Read the model definition and answer for the solid it produces. Units are mm, in the model's axes. Face numbers are marked on the shaded views. A direction names the side the tool comes from. Coordinates: 2 decimals unless noted, no trailing zeros. Loops run counter-clockwise (first coordinate to the right, second up) from the corner with the lowest first, then second, coordinate; pieces in that order, holes last. Notation, with made-up numbers: (-25.75, 73.5) -> (8.25, 73.5) arc R14 cw to (8.25, 88.5) -> close; hole circle Ø7 at (43.25, 34.5). An arc over 180 degrees is marked (long way). Answer as a JSON object with one key per item and string values. Group by question number.
1) Which of the six approach directions +Z, -Z, +X, -X, +Y, -Y give full straight-line access (tool end or side, diameter ignored) to the marked faces 1 and 2?
2) Section A-A, the plane y = 0 is taken. Give the vertices of the cut face in (x, z) (3 decimals).
3) Consider probe 1 along Y at (x, z) = (0, -7.9) (3 decimals); probe 2 along X at (y, z) = (1, -47); probe 3 along Z at (x, y) = (-46, -65). Determine where each line is inside the solid, lowest interval first. Write a range as [from, to].
4) Flat-ended cylindrical pins translate along their axes: P1, Ø10, axis at y = -51.5, z = -10.5, coming from the +X side; P2, Ø10, axis at x = 67, z = -30.5, coming from the -Y side; P3, Ø4, axis at y = 41.5, z = -35, coming from the -X side. Find the tip coordinate at first contact, or state that the pin passes through.
5) Section C-C, the plane z = -15 is taken. Give the vertices of the cut face in (x, y).
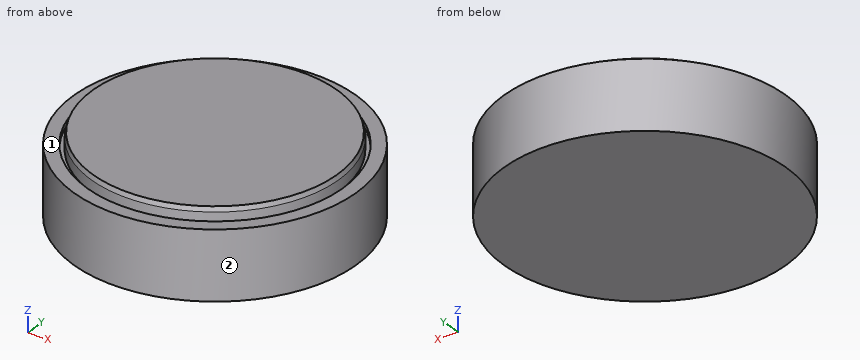
from build123d import *

# Parameters (mm, degrees)
F2_SIZE2 = 3
F2_SIZE  = 0.8038475773
F3_W     = 2.715
F3_H     = 3


with BuildPart() as f1:
    # F0 (on Front) → F1 (revolve)
    with BuildSketch(Plane.XZ):
        Polygon((77.785, 0), (0, 0), (0, -50), (88.9, -50), (88.9, -7), (77.785, -7), align=None)
    revolve(axis=Axis((0, 0, -25), (0, 0, 1)))

    # F2
    f2_edges = [f1.edges().sort_by_distance(p)[0] for p in [
        (-77.785, 0, 0),
    ]]
    f2_side = f1.faces().sort_by_distance((0, 0, 0))[0]
    chamfer(f2_edges, length=F2_SIZE, length2=F2_SIZE2, reference=f2_side)

    # F3 (on Front) → F4 (revolve, cut)
    with BuildSketch(Plane.XZ):
        with Locations((79.1425, -8.5)):
            Rectangle(F3_W, F3_H)
    revolve(axis=Axis((0, 0, -8.4670595825), (0, 0, 1)), mode=Mode.SUBTRACT)


solid = f1.part
Determined:
{
 "1": {"face 1": "+Z", "face 2": "+Z, -Z"},
 "2": {"outline": "(-88.9, -50) -> (88.9, -50) -> (88.9, -7) -> (80.5, -7) -> (80.5, -10) -> (77.785, -10) -> (77.785, -3) -> (76.981, 0) -> (-76.981, 0) -> (-77.785, -3) -> (-77.785, -10) -> (-80.5, -10) -> (-80.5, -7) -> (-88.9, -7) -> close"},
 "3": {"probe 1": "[-88.9, -80.5], [-77.785, 77.785], [80.5, 88.9]", "probe 2": "[-88.89, 88.89]", "probe 3": "[-50, -10]"},
 "4": {"P1": "x = 75.77", "P2": "y = -63.71", "P3": "x = -79.64"},
 "5": {"outline": "circle Ø177.8 at (0, 0)"}
}
